Autodesk Inventor part; units mm, degrees
ref_plane "YZ Plane" through (0, 0, 0) normal (1, 0, 0) x (0, 1, 0)
ref_plane "XZ Plane" through (0, 0, 0) normal (0, 1, 0) x (-1, 0, 0)
ref_plane "XY Plane" through (0, 0, 0) normal (0, 0, 1) x (1, 0, 0)
sketch "Sketch1" plane through (0, 0, 0) normal (0, 0, 1) x (1, 0, 0)
  line L0 (0, 0) -> (-25.4, 0)
  line L1 (-25.4, 0) -> (-25.4, 25.4)
  line L2 (-25.4, 25.4) -> (0, 25.4)
  line L3 (0, 25.4) -> (0, 0)
  line L4 (-3.175, 22.225) -> (-22.225, 22.225)
  line L5 (-22.225, 22.225) -> (-22.225, 3.175)
  line L6 (-22.225, 3.175) -> (-3.175, 3.175)
  line L7 (-3.175, 3.175) -> (-3.175, 22.225)
  dimension "d0" = 25.4
  dimension "d2" = 25.4
  dimension "d3" = 3.175
extrude "Extrusion1" add sketch "Sketch1" along normal blind 190.5
sketch "Sketch2" plane through (-25.4, 25.4, 0) normal (0, 1, 0) x (1, 0, 0)
  circle A0 centre (12.7, -19.05) radius 3.3782
  circle A1 centre (12.7, -6.35) radius 3.3782
extrude "Extrusion2" cut sketch "Sketch2" against normal blind 25.4
sketch "Sketch3" plane through (-25.4, 25.4, 0) normal (0, 1, 0) x (1, 0, 0)
  circle A0 centre (12.7, -203.2) radius 3.3782
  circle A1 centre (12.7, -177.8) radius 3.3782
extrude "Extrusion3" cut sketch "Sketch3" against normal blind 25.4
sketch "Sketch4" plane through (-25.4, 25.4, 0) normal (0, 1, 0) x (1, 0, 0)
  circle A0 centre (12.7, -63.5) radius 3.3782
  circle A1 centre (12.7, -88.9) radius 3.3782
extrude "Extrusion4" cut sketch "Sketch4" against normal blind 25.4
properties part number "p80 mount" material "Aluminum 6061"
Check sheet for the modelled part. Datum: model origin and axes. Units: mm. A direction names the side the tool comes from. Give positions to 0.01 mm unless a question says otherwise; leave off trailing zeros. Order: outer loops, then holes, each group sorted by start corner. A loop starts at its lowest first (then second) coordinate and runs counter-clockwise, first axis right, second up. Notation, with made-up numbers: M 0,-7.75 L 5,-7.75 A20 cw 5,27.25 Z; hole C 37.25,7 d6. An arc over 180 degrees is marked long. Answer as CSV lines item,"result". Start each with the question number.
Item 1: Thickness scan on line 1 (Z direction, x = -12.7, y = 24.45); line 2 (X direction, y = 12.5, z = 90.5) (3 decimals); line 3 (Y direction, x = -6.25, z = 168) (3 decimals). Record the ranges inside material, lowest first. Write a range as [from, to].
Item 2: Cross-section at C-C on z = 142. Enter the section's corners in (x, y) (3 decimals), plus the area to 3 significant figures.
Item 3: Cross-section at B-B on x = -7.5. Enter the section's corners in (y, z) (3 decimals), plus the area to 3 significant figures.
Item 4: Cross-section at A-A on z = 88.9. Enter the section's corners in (x, y) (3 decimals), plus the area to 3 significant figures.
Item 5: Mould release check, pull along Z, two halves, no side actions. Record for faces 1 (the face through (-2, 13, 190.5)), 2 (the face through (-13.14, 1.61, 85.55)), 3 (the face through (-13, 22.225, 94)): +Z half, -Z half, draft (parallel to the pull), parting line (faces both ways), or undercut.
Item 6: Tool access check on faces 4 (the face through (-15.19, 1.61, 4.067)), 5 (the face through (-13, 3.175, 94)). Record the directions out of +Z, -Z, +X, -X, +Y, -Y that give a thin tool (end or side, any length) a straight path to the whole face; none if there is none.
Established:
1,line 1,"z = [0, 2.97], [9.73, 15.67], [22.43, 60.12], [66.88, 85.52], [92.28, 174.42], [181.18, 190.5]"
1,line 2,"x = [-25.4, -22.225], [-3.175, 0]"
1,line 3,"y = [0, 3.175], [22.225, 25.4]"
2,outline,"M -25.4,0 L 0,0 L 0,25.4 L -25.4,25.4 Z; hole M -22.225,3.175 L -3.175,3.175 L -3.175,22.225 L -22.225,22.225 Z"
2,area,"282 mm^2"
3,outline,"M 0,0 L 3.175,0 L 3.175,190.5 L 0,190.5 Z; M 22.225,0 L 25.4,0 L 25.4,190.5 L 22.225,190.5 Z"
3,area,"1,210 mm^2"
4,outline,"M -25.4,0 L -16.078,0 L -16.078,3.175 L -22.225,3.175 L -22.225,22.225 L -16.078,22.225 L -16.078,25.4 L -25.4,25.4 Z; M -9.322,0 L 0,0 L 0,25.4 L -9.322,25.4 L -9.322,22.225 L -3.175,22.225 L -3.175,3.175 L -9.322,3.175 Z"
4,area,"239 mm^2"
5,face 1,"+Z half"
5,face 2,"undercut"
5,face 3,"draft"
6,face 4,"+Y, -Y"
6,face 5,"+Z, -Z"
